Geometry check sheet. Reference: the model listing, model coordinates, mm. A direction names the side the tool comes from. Give positions to 0.01 mm unless a question says otherwise; leave off trailing zeros. Order: outer loops, then holes, each group sorted by start corner. A loop starts at its lowest first (then second) coordinate and runs counter-clockwise, first axis right, second up. Notation, with made-up numbers: M -5.5,52 L 18.5,52 A13 cw 18.5,63 Z; hole C 64.5,7 d8. An arc over 180 degrees is marked long. Answer as CSV lines item,"result". Start each with the question number.
```python
from build123d import *

# Parameters (mm, degrees)
F0_W     = 59.02
F0_H     = 20.92
F0_W_2   = 48.86
F0_H_2   = 10.76
F1_DEPTH = 22.86
F2_W     = 59.02
F2_H     = 7.62
F2_R     = 2.6035
F3_DEPTH = 5.08
F4_W     = 41.24
F4_H     = 5.08
F5_DEPTH = 22.861


with BuildPart() as f1:
    # F0 (on Top) → F1 (new body)
    with BuildSketch(Plane.XY):
        Rectangle(F0_W, F0_H)
        Rectangle(F0_W_2, F0_H_2, mode=Mode.SUBTRACT)
    extrude(amount=F1_DEPTH)

    # F2 (on face) → F3 (join)
    with BuildSketch(Plane.XY.offset(22.86)):
        with Locations((0, 14.27)):
            Rectangle(F2_W, F2_H)
        with Locations((0, 13.635)):
            Circle(F2_R, mode=Mode.SUBTRACT)
    extrude(amount=-F3_DEPTH)

    # F4 (on face) → F5 (cut, through all)
    with BuildSketch(Plane(origin=(0, 0, 0), x_dir=(1, 0, 0), z_dir=(0, 0, -1))):
        with Locations((0, 7.92)):
            Rectangle(F4_W, F4_H)
    extrude(amount=-F5_DEPTH, mode=Mode.SUBTRACT)


solid = f1.part
```
Item 1: Access from +Z, -Z, +X, -X, +Y, -Y to the whole of each face (thin tool, end or side, straight path). Record for faces 1 (the face through (0, 17, 17.78)), 2 (the face through (24.43, 0, 11)), 3 (the face through (-20.62, -8, 11)).
Item 2: Scan lines: line 1 along X through (y, z) = (-0.25, 13); line 2 along Y through (x, z) = (0, 20.55); line 3 along X through (y, z) = (-5.5, 21.5). Record each from-to range of solid material in increasing order.
Item 3: Section check D-D on x = 6.5. Record the boundary of the cut face in (y, z), then the cut area to 3 significant figures.
Item 4: Section check C-C on z = 6.5. Record the boundary of the cut face in (x, y).
Item 5: Section check A-A on x = 0. Record the boundary of the cut face in (y, z).
Item 6: Depth check by flat-ended pin: pin 1 Ø2 at (x, y) = (23.5, -3.5) entering from -Z; pin 2 Ø1 at (x, z) = (-18, 5) entering from -Y; pin 3 Ø4 at (x, y) = (3, 15.5) entering from -Z; pin 4 Ø1.1 at (x, z) = (22.5, 10) entering from +Y. Enter the tip coordinate at first touch or a pass-through.
Item 7: Draft check along X on faces 4 (the face through (22, -5.38, 11)), 5 (the face through (20.62, -8, 11)), 6 (the face through (29.51, 0, 12)), 7 (the face through (0, 18.08, 20)). Enter one of: pulls with the +X half, pulls with the -X half, needs draft (parallel to the pull), parting line crosses it, or undercut.
Item 8: Section check B-B on y = -4.5. Record the boundary of the cut face in (x, z), then the cut area to 3 significant figures.
Numbers:
1,face 1,"-Z, +X, -X, +Y"
1,face 2,"+Z, -Z"
1,face 3,"+Z, -Z, -Y"
2,line 1,"-29.51 to -24.43, 24.43 to 29.51"
2,line 2,"5.38 to 11.03, 16.24 to 18.08"
2,line 3,"-29.51 to -20.62, 20.62 to 29.51"
3,outline,"M 5.38,0 L 10.46,0 L 10.46,17.78 L 18.08,17.78 L 18.08,22.86 L 5.38,22.86 Z"
3,area,"155 mm2"
4,outline,"M -29.51,-10.46 L -20.62,-10.46 L -20.62,-5.38 L -24.43,-5.38 L -24.43,5.38 L 24.43,5.38 L 24.43,-5.38 L 20.62,-5.38 L 20.62,-10.46 L 29.51,-10.46 L 29.51,10.46 L -29.51,10.46 Z"
5,outline,"M 5.38,0 L 10.46,0 L 10.46,17.78 L 11.03,17.78 L 11.03,22.86 L 5.38,22.86 Z; M 16.24,17.78 L 18.08,17.78 L 18.08,22.86 L 16.24,22.86 Z"
6,pin 1,"z = 0"
6,pin 2,"y = 5.38"
6,pin 3,"z = 17.78"
6,pin 4,"y = 10.46"
7,face 4,"undercut"
7,face 5,"undercut"
7,face 6,"pulls with the +X half"
7,face 7,"needs draft"
8,outline,"M -29.51,0 L -24.43,0 L -24.43,22.86 L -29.51,22.86 Z; M 24.43,0 L 29.51,0 L 29.51,22.86 L 24.43,22.86 Z"
8,area,"232 mm2"
